Could you check a few things on this model? Use its own coordinates, in mm. Give positions to 0.01 mm unless a question says otherwise; leave off trailing zeros. Order: outer loops, then holes, each group sorted by start corner. A loop starts at its lowest first (then second) coordinate and runs counter-clockwise, first axis right, second up.
(1) If I drill on probe 1 along Y at (x, z) = (-130.5, 52); probe 2 along X at (y, z) = (408, -81); probe 3 along Y at (x, z) = (59, 68.5), over which ranges is the centre line in solid material (lowest first)?
(2) Will these pins go through, and if not, where does the flat tip stop? pin 1 (1.5 mm diameter, centred on x = -78, z = 66, fed in from +Y); pin 2 (6 mm diameter, centred on x = -65.5, y = 586, fed in from -Z); pin 3 (1.6 mm diameter, centred on x = -39, z = 72.5, fed in from +Y); pin 4 (3 mm diameter, centred on x = 40.5, z = 78, fed in from +Y).
(3) Imagine slicing it at B-B, the plane z = 59. Write out the boundary of the cut face in (x, y), then the cut area to 3 significant figures.
(4) Imagine slicing it at A-A, the plane x = -74. Write out the boundary of the cut face in (y, z), then the cut area to 3 significant figures.
(5) Imagine slicing it at C-C, the plane y = 682. Write out the boundary of the cut face in (x, z), then the cut area to 3 significant figures.
(6) Imagine slicing it at D-D, the plane y = 448. Write out the boundary of the cut face in (x, z).
from build123d import *

# Parameters (mm, degrees)
SKETCH1_W           = 300
SKETCH1_H           = 200
BOSS_EXTRUDE1_DEPTH = 25.4
SKETCH2_W           = 200
SKETCH2_H           = 150
CUT_EXTRUDE1_DEPTH  = 25.4
SKETCH3_W           = 25
SKETCH3_H           = 50
BOSS_EXTRUDE2_DEPTH = 724.6
SKETCH5_W           = 25
SKETCH5_H           = 25
BOSS_EXTRUDE3_DEPTH = 100
SKETCH6_W           = 25
SKETCH6_H           = 25
BOSS_EXTRUDE4_DEPTH = 150
SKETCH7_W           = 300
SKETCH7_H           = 25
BOSS_EXTRUDE5_DEPTH = 25
SKETCH8_W           = 300
SKETCH8_H           = 19.64917274
CUT_EXTRUDE2_DEPTH  = 5
FILLET1_R           = 10


with BuildPart() as part:
    # Sketch1 → Boss-Extrude1 (new body)
    with BuildSketch(Plane(origin=(0, 0, 0), x_dir=(1, 0, 0), z_dir=(0, 1, 0))):
        Rectangle(SKETCH1_W, SKETCH1_H)
    extrude(amount=BOSS_EXTRUDE1_DEPTH)

    # Sketch2 → Cut-Extrude1 (cut)
    with BuildSketch(Plane(origin=(0, 25.4, 0), x_dir=(1, 0, 0), z_dir=(0, 1, 0))):
        with Locations((0, -25)):
            Rectangle(SKETCH2_W, SKETCH2_H)
    extrude(amount=-CUT_EXTRUDE1_DEPTH, mode=Mode.SUBTRACT)

    # Sketch3 → Boss-Extrude2 (add)
    with BuildSketch(Plane(origin=(0, 25.4, 0), x_dir=(1, 0, 0), z_dir=(0, 1, 0))):
        with Locations((0, 75)):
            Rectangle(SKETCH3_W, SKETCH3_H)
    extrude(amount=BOSS_EXTRUDE2_DEPTH)

    # Sketch5 → Boss-Extrude3 (add)
    with BuildSketch(Plane.XY.offset(-50)):
        with Locations((0, 737.5)):
            Rectangle(SKETCH5_W, SKETCH5_H)
    extrude(amount=BOSS_EXTRUDE3_DEPTH)

    # Sketch6 → Boss-Extrude4 (add)
    with BuildSketch(Plane.XZ.offset(-725)):
        with Locations((0, 37.5)):
            Rectangle(SKETCH6_W, SKETCH6_H)
    extrude(amount=BOSS_EXTRUDE4_DEPTH)

    # Sketch7 → Boss-Extrude5 (add)
    with BuildSketch(Plane.XY.offset(50)):
        with Locations((0, 587.5)):
            Rectangle(SKETCH7_W, SKETCH7_H)
    extrude(amount=BOSS_EXTRUDE5_DEPTH)

    # Sketch8 → Cut-Extrude2 (cut)
    with BuildSketch(Plane(origin=(0, 600, 0), x_dir=(1, 0, 0), z_dir=(0, 1, 0))):
        with Locations((0, -59.82458637)):
            Rectangle(SKETCH8_W, SKETCH8_H)
    extrude(amount=-CUT_EXTRUDE2_DEPTH, mode=Mode.SUBTRACT)

    # Fillet1
    fillet1_edges = [part.edges().sort_by_distance(p)[0] for p in [
        (-150, 25.4, 0),
        (-100, 0, 25),
        (0, 0, -50),
        (100, 0, 25),
        (-100, 25.4, 25),
        (100, 25.4, 25),
        (-81.25, 25.4, -100),
        (12.5, 387.7, -100),
        (-12.5, 387.7, -100),
        (12.5, 750, -25),
        (-12.5, 750, -25),
        (-12.5, 375.2, -50),
        (12.5, 375.2, -50),
        (150, 25.4, 0),
        (-150, 0, 0),
        (0, 0, -100),
        (-12.5, 650, 25),
        (12.5, 650, 25),
        (150, 0, 0),
        (81.25, 25.4, -100),
    ]]
    fillet(fillet1_edges, radius=FILLET1_R)


solid = part.part
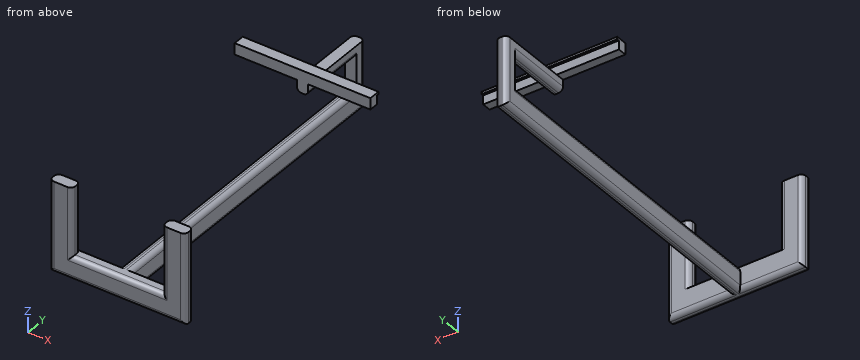
Answer block:
1. probe 1: y = 0 to 25.4, 575 to 595
1. probe 2: x = -12.5 to 12.5
1. probe 3: y = 575 to 595
2. pin 1: stops at y = 595
2. pin 2: stops at z = 50
2. pin 3: stops at y = 600
2. pin 4: passes through
3. outline: (-150, 10) arc R10 ccw to (-140, 0) - (-110, 0) arc R10 ccw to (-100, 10) - (-100, 15.4) arc R10 ccw to (-110, 25.4) - (-140, 25.4) arc R10 ccw to (-150, 15.4) - close; (-150, 575) - (150, 575) - (150, 595) - (-150, 595) - close; (100, 10) arc R10 ccw to (110, 0) - (140, 0) arc R10 ccw to (150, 10) - (150, 15.4) arc R10 ccw to (140, 25.4) - (110, 25.4) arc R10 ccw to (100, 15.4) - close
3. area: 8,370 mm2
4. outline: (0, -90) arc R10 ccw to (10, -100) - (15.4, -100) arc R10 ccw to (25.4, -90) - (25.4, -50) - (10, -50) arc R10 ccw to (0, -60) - close; (575, 50) - (595, 50) - (595, 69.65) - (600, 69.65) - (600, 75) - (575, 75) - close
4. area: 1,730 mm2
5. outline: (-12.5, -90) arc R10 ccw to (-2.5, -100) - (2.5, -100) arc R10 ccw to (12.5, -90) - (12.5, -60) arc R10 ccw to (2.5, -50) - (-2.5, -50) arc R10 ccw to (-12.5, -60) - close; (-12.5, 35) arc R10 ccw to (-2.5, 25) - (2.5, 25) arc R10 ccw to (12.5, 35) - (12.5, 50) - (-12.5, 50) - close
5. area: 1,750 mm2
6. outline: (-12.5, -90) arc R10 ccw to (-2.5, -100) - (2.5, -100) arc R10 ccw to (12.5, -90) - (12.5, -60) arc R10 ccw to (2.5, -50) - (-2.5, -50) arc R10 ccw to (-12.5, -60) - close
